Here's how the part is built. I have some questions about the finished solid (model axes, mm). Coordinates: 2 decimals unless noted, no trailing zeros. Write each loop counter-clockwise with the first axis right and the second up, starting at its lowest first coordinate (ties: lowest second). Pieces come first, ordered by that corner, then holes. Notation, with made-up numbers: (53, -37.5) -> (86, -37.5) arc R29 cw to (86, -2.5) -> close; hole circle Ø10 at (-35.5, 58). An arc over 180 degrees is marked (long way). Put each result on its own line as item: value.
```python
from build123d import *

# Parameters (mm, degrees)
EXTRUDE_1_DEPTH = 5
FILLET_1_R      = 0.5


with BuildPart() as part:
    # Эскиз1 → Бобышка-Вытянуть1 (new body)
    with BuildSketch(Plane(origin=(0, 0, 0), x_dir=(1, 0, 0), z_dir=(0, 1, 0))):
        with BuildLine():
            Line((-25.434053198, 5.944166553), (-25.839949009, 5.944166553))
            ThreePointArc((-25.839949009, 5.944166553), (-27.213842529, 6.49075106), (-27.836787137, 7.831749958))
            ThreePointArc((-27.836787137, 7.831749958), (-10.907888473, 50.216792744), (32.43979713, 64.501666381))
            ThreePointArc((32.43979713, 64.501666381), (34.329532824, 63.515149683), (35.086918855, 61.522492515))
            Line((35.086918855, 61.522492515), (35.086918855, 59.843935519))
            ThreePointArc((35.086918855, 59.843935519), (34.242597527, 57.757539233), (32.184885879, 56.845535535))
            ThreePointArc((32.184885879, 56.845535535), (-4.499436157, 42.261590709), (-23.458092531, 7.635007302))
            ThreePointArc((-23.458092531, 7.635007302), (-24.133729873, 6.424574749), (-25.434053198, 5.944166553))
        make_face()
    extrude(amount=EXTRUDE_1_DEPTH)

    # Скругление1
    fillet_1_edges = [part.edges().sort_by_distance(p)[0] for p in [
        (34.329532824, 5, -63.515149683),
        (-10.907888473, 5, -50.216792744),
        (-27.213842529, 5, -6.49075106),
        (-25.637001104, 5, -5.944166553),
        (-24.133729873, 5, -6.424574749),
        (-4.499436157, 5, -42.261590709),
        (34.242597527, 5, -57.757539233),
        (35.086918855, 5, -60.683214017),
    ]]
    fillet(fillet_1_edges, radius=FILLET_1_R)


solid = part.part
```
Item 1: Please list where these lines run through material, in increasing order: line 1 along Z through (x, y) = (22, 0.7); line 2 along X through (y, z) = (1.2, -34); line 3 along Z through (x, y) = (23, 2.75). Write a range as from..to.
Output:
line 1: z = -64.72..-55.61
line 2: x = -22.72..-12.19
line 3: z = -64.79..-55.81
Item 2: For P1, Ø12, axis at x = -3.5, z = -40.5, coming from the -Y side; P2, Ø1.5, axis at y = 4, z = -50.5, coming from the +X side; P3, Ø2, axis at y = 1.5, z = -45.5, coming from the -X side, each with a flat end and sliding along its axis, tell me the tip position at first contact or that it passes through.
Output:
P1: stops at y = 0
P2: stops at x = 9.11
P3: stops at x = -16.17
Item 3: Imagine slicing it at A-A on y = 2.5. Write out the boundary of the cut face in (x, z) (1 decimal).
Output:
outline: (-27.8, -7.8) arc R54 ccw to (32.4, -64.5) arc R3 ccw to (35.1, -61.5) -> (35.1, -59.8) arc R3 ccw to (32.2, -56.8) arc R58.2 cw to (-23.5, -7.6) arc R2 ccw to (-25.4, -5.9) -> (-25.8, -5.9) arc R2 ccw to start
